Answer from the drawing. Dimensions are ordinates in mm from the lowest x, y and z of the part. A direction names the side the tool comes from. Round coordinates to 2 decimals unless told otherwise and drop trailing zeros. Write each loop counter-clockwise with the first axis right and the second up, starting at its lowest first coordinate (ties: lowest second). Pieces come first, ordered by that corner, then holes. Notation, with made-up numbers: (-17.5, 43) - (-11.5, 43) arc R22 ccw to (-11.5, 62) - close; hole circle Ø11 at (-5, 6). An arc over 180 degrees is marked (long way). Use a Markdown table: item, result. Add a question column.
1) A tool of negligible diameter and unlimited length cuts with its end or side. For the marked faces 4 and 5, from which of +Z, -Z, +X, -X, +Y, -Y can it reach the whole face along a straight path? Write none if from no direction.
2) A cutting plane is placed at C-C (y = 15.5). Give the vertices of the cut face in (x, z) (3 decimals), then the cut area to 3 significant figures.
3) A cutting plane is placed at D-D (x = 21.5). Give the vertices of the cut face in (y, z) (3 decimals).
4) A cutting plane is placed at B-B (z = 13.5). Give the vertices of the cut face in (x, y) (3 decimals), then the cut area to 3 significant figures.
5) A cutting plane is placed at A-A (x = 12.7). Give the vertices of the cut face in (y, z) (3 decimals), then the cut area to 3 significant figures.
6) Find the intervals of material crossed by probe 1 along Y at (x, z) = (12.7, 1.55) (3 decimals); probe 2 along Z at (x, y) = (12.7, 1.8) (3 decimals); probe 3 along Z at (x, y) = (19.25, 21.5) (3 decimals), in increasing order. Write a range as from..to.
7) Determine the mould class of the marked faces 1, 2 and 3 for opening direction Y: +Y half, -Y half, draft (parallel to the pull), parting line (faces both ways), or undercut.
8) Each of these flat-tipped pins is pushed along its axis until it touches: P1, Ø3, axis at x = 22, z = 22, coming from the +Y side (3 decimals); P2, Ø10, axis at x = 12.7, y = 15.875, coming from the +Z side; P3, Ø6.5, axis at x = 10, y = 19.5, coming from the +Z side (3 decimals). Where does it stop, or does it pass through?
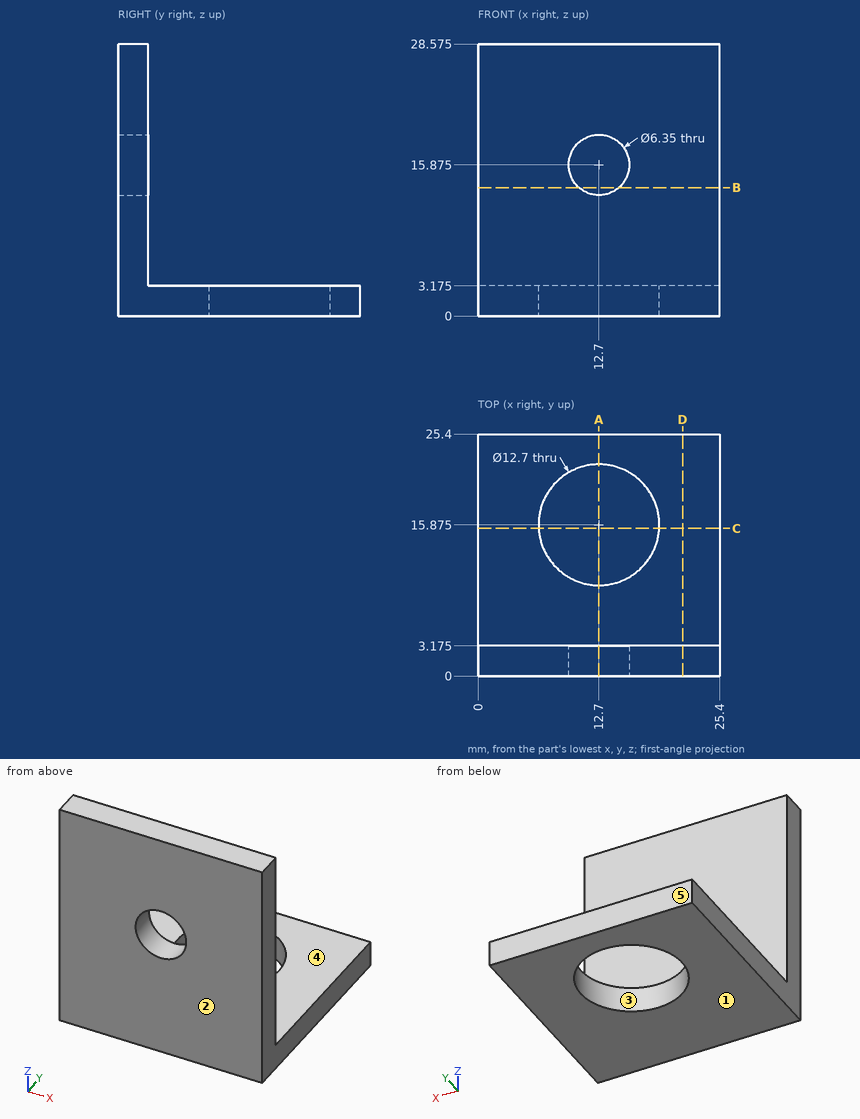
Entries:
| question | item | result |
|---|---|---|
| 1 | face 4 | +Z, +X, -X, +Y |
| 1 | face 5 | +Z, -Z, +X, -X, +Y |
| 2 | outline | (0, 0) - (6.361, 0) - (6.361, 3.175) - (0, 3.175) - close; (19.039, 0) - (25.4, 0) - (25.4, 3.175) - (19.039, 3.175) - close |
| 2 | area | 40.4 mm² |
| 3 | outline | (0, 0) - (25.4, 0) - (25.4, 3.175) - (3.175, 3.175) - (3.175, 28.575) - (0, 28.575) - close |
| 4 | outline | (0, 0) - (10.593, 0) - (10.593, 3.175) - (0, 3.175) - close; (14.807, 0) - (25.4, 0) - (25.4, 3.175) - (14.807, 3.175) - close |
| 4 | area | 67.3 mm² |
| 5 | outline | (0, 0) - (9.525, 0) - (9.525, 3.175) - (3.175, 3.175) - (3.175, 12.7) - (0, 12.7) - close; (0, 19.05) - (3.175, 19.05) - (3.175, 28.575) - (0, 28.575) - close; (22.225, 0) - (25.4, 0) - (25.4, 3.175) - (22.225, 3.175) - close |
| 5 | area | 101 mm² |
| 6 | probe 1 | y = 0..9.525, 22.225..25.4 |
| 6 | probe 2 | z = 0..12.7, 19.05..28.575 |
| 6 | probe 3 | z = 0..3.175 |
| 7 | face 1 | draft |
| 7 | face 2 | -Y half |
| 7 | face 3 | undercut |
| 8 | P1 | stops at y = 3.175 |
| 8 | P2 | passes through |
| 8 | P3 | stops at z = 3.175 |
